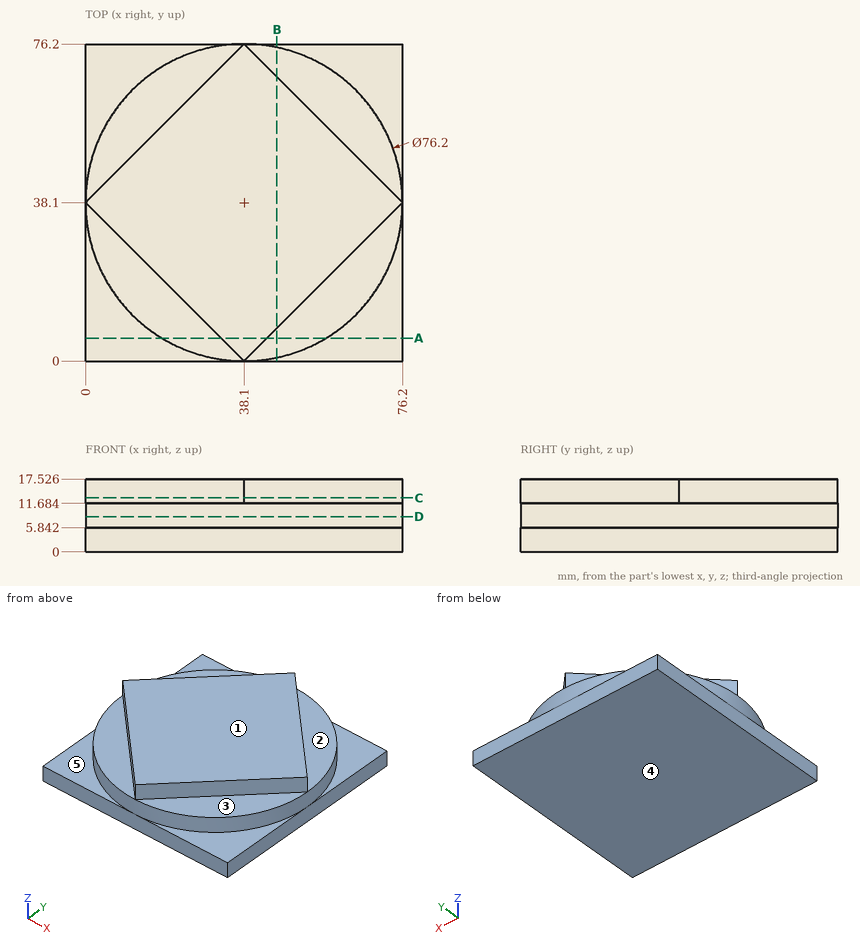
Input: dimensioned drawing with shaded views. Units: mm. Origin: part minimum x, y, z. A direction names the side the tool comes from. Coordinates: 2 decimals unless noted, no trailing zeros. Loops run counter-clockwise (first coordinate to the right, second up) from the corner with the lowest first, then second, coordinate; pieces in that order, holes last. Notation, with made-up numbers: M 54.5,48 L 98.5,48 A32 cw 98.5,83 Z; hole C 21,35 d4. An arc over 180 degrees is marked long. One line per item, written item: value.
(1) Section C-C (z = 13). Output: boundary loops of the cut face in (x, y), and give its area (3 significant figures).
Filled in:
outline: M 0,38.1 L 38.1,0 L 76.2,38.1 L 38.1,76.2 Z
area: 2,900 mm^2
(2) Section B-B (x = 46). Output: boundary loops of the cut face in (y, z).
Filled in:
outline: M 0,0 L 76.2,0 L 76.2,5.84 L 75.37,5.84 L 75.37,11.68 L 68.3,11.68 L 68.3,17.53 L 7.9,17.53 L 7.9,11.68 L 0.83,11.68 L 0.83,5.84 L 0,5.84 Z
(3) Section D-D (z = 8.5). Output: boundary loops of the cut face in (x, y), and give its area (3 significant figures).
Filled in:
outline: C 38.1,38.1 d76.2
area: 4,560 mm^2
(4) Reachability of the marked faces 1, 2, 3, 4 and 5 from +Z, -Z, +X, -X, +Y, -Y: full face, straight path, thin tool, end or side. Return the list, or none.
Filled in:
face 1: +Z, +X, -X, +Y, -Y
face 2: +Z, +X, +Y
face 3: +Z, +X, -Y
face 4: -Z, +X, -X, +Y, -Y
face 5: +Z, -X, -Y
(5) Pin query (flat end, axial travel): pin 1 (2 mm diameter, centred on x = 11.5, y = 62, fed in from +Z); pin 2 (1.5 mm diameter, centred on x = 11, z = 11.5, fed in from -Y); pin 3 (1.5 mm diameter, centred on y = 50, z = 13, fed in from +X). Return the tip coordinate at first contact, or that it passes through.
Filled in:
pin 1: z = 11.68
pin 2: y = 10.58
pin 3: x = 65.05
(6) Line query: line 1 along Z through (x, y) = (60.5, 67); line 2 along Y through (x, z) = (10.5, 11) (3 decimals); line 3 along X through (y, z) = (42.5, 15.5). Output: solid intervals per line, ascending. Write a range as from..to.
Filled in:
line 1: 0..11.68
line 2: 11.835..64.365
line 3: 4.4..71.8
(7) Section A-A (y = 5.5). Output: boundary loops of the cut face in (x, z).
Filled in:
outline: M 0,0 L 76.2,0 L 76.2,5.84 L 57.82,5.84 L 57.82,11.68 L 43.6,11.68 L 43.6,17.53 L 32.6,17.53 L 32.6,11.68 L 18.38,11.68 L 18.38,5.84 L 0,5.84 Z
